Source: CAD feature listing. Evaluate the final solid. Frame: model axes, mm. A direction names the side the tool comes from. Round coordinates to 2 decimals unless told otherwise and drop trailing zeros. Write each loop counter-clockwise with the first axis right and the second up, starting at its lowest first coordinate (ties: lowest second). Pieces come first, ordered by that corner, then holes.
from build123d import *

# Parameters (mm, degrees)
PAD_DEPTH = 100


with BuildPart() as part:
    # Sketch → Pad (new body)
    with BuildSketch(Plane.XY):
        with BuildLine():
            Line((50, 0), (0, 0))
            Line((0, 0), (25, 43.30127))
            Line((25, 43.30127), (45, 8.660254))
            Line((45, 8.660254), (51.928203, 12.660254))
            Line((51.928203, 12.660254), (48.928203, 17.856406))
            Line((48.928203, 17.856406), (51.526279, 19.356406))
            Line((51.526279, 19.356406), (56.026279, 11.562178))
            Line((56.026279, 11.562178), (43.901924, 4.562178))
            Line((33.660254, 22.30127), (43.901924, 4.562178))
            ThreePointArc((33.660254, 22.30127), (25, 27.30127), (16.339746, 22.30127))
            Line((13.856406, 18), (16.339746, 22.30127))
            ThreePointArc((13.856406, 18), (13.856406, 8), (22.51666, 3))
            Line((22.51666, 3), (50, 3))
            Line((50, 3), (50, 0))
        make_face()
    extrude(amount=PAD_DEPTH)


solid = part.part
1) Contact query for flat-ended pins moving along their axis: P1, Ø6, axis at y = 24, z = 82.5, coming from the +X side; P2, Ø2, axis at x = 36.5, z = 68, coming from the +Y side; P3, Ø3.5, axis at y = 2, z = 54, coming from the +X side. Output: stop coordinate, or through.
Taken from the geometry:
P1: stops at x = 37.88
P2: stops at y = 25.11
P3: stops at x = 50
2) Section query D-D on y = 26. Return the cut outline in (x, z).
Taken from the geometry:
outline: (15.01, 0) - (20.07, 0) - (20.07, 100) - (15.01, 100) - close; (29.93, 0) - (34.99, 0) - (34.99, 100) - (29.93, 100) - close
3) Material intervals for line 1 (X direction, y = 11, z = 55); line 2 (X direction, y = 13.5, z = 95); line 3 (Y direction, x = 45.5, z = 51), sorted ascending.
Taken from the geometry:
line 1: x = 6.35 to 12.72, 40.19 to 43.65, 49.05 to 55.05
line 2: x = 7.79 to 12.53, 38.74 to 42.21, 51.44 to 54.91
line 3: y = 0 to 3, 5.48 to 8.95
4) Pull-direction query (X, two-part tool) for faces 1 (the face through (34.4, 21.8, 0)), 2 (the face through (34.86, 26.22, 49.3)), 3 (the face through (25.1, 27.3, 49.3)), 4 (the face through (50.05, 8.11, 49.3)); classes: released by +X, released by -X, zero draft, split by the parting line, or undercut.
Taken from the geometry:
face 1: zero draft
face 2: undercut
face 3: undercut
face 4: released by +X
5) Section query C-C on y = 15. Return the cut outline in (x, z), then the cut area to 3 significant figures.
Taken from the geometry:
outline: (8.66, 0) - (12.72, 0) - (12.72, 100) - (8.66, 100) - close; (37.88, 0) - (41.34, 0) - (41.34, 100) - (37.88, 100) - close; (50.58, 0) - (54.04, 0) - (54.04, 100) - (50.58, 100) - close
area: 1,100 mm2
6) Section query B-B on z = 36. Return the cut outline in (x, y).
Taken from the geometry:
outline: (0, 0) - (50, 0) - (50, 3) - (22.52, 3) arc R10 cw to (13.86, 18) - (16.34, 22.3) arc R10 cw to (33.66, 22.3) - (43.9, 4.56) - (56.03, 11.56) - (51.53, 19.36) - (48.93, 17.86) - (51.93, 12.66) - (45, 8.66) - (25, 43.3) - close
7) Section query A-A on x = 42. Return the cut outline in (y, z), then the cut area to 3 significant figures.
Taken from the geometry:
outline: (0, 0) - (3, 0) - (3, 100) - (0, 100) - close; (7.86, 0) - (13.86, 0) - (13.86, 100) - (7.86, 100) - close
area: 900 mm2
8) Reachability of faces 5 (the face through (50.45, 15.22, 49.3)), 6 (the face through (50, 2, 49)), 7 (the face through (50.209, 18.596, 49.3)), 8 (the face through (36, 3, 49)) from +Z, -Z, +X, -X, +Y, -Y: full face, straight path, thin tool, end or side. Return the list, or none.
Taken from the geometry:
face 5: +Z, -Z
face 6: +Z, -Z, +X, -Y
face 7: +Z, -Z, +Y
face 8: +Z, -Z, +X
